from build123d import *

# Parameters (mm, degrees)
SKETCH1_R             = 22.5
BOSS_EXTRUDE1_DEPTH   = 75
BOSS_EXTRUDE1_2_DEPTH = 75
SKETCH1_W             = 45
SKETCH1_H             = 45
BOSS_EXTRUDE1_3_DEPTH = 75
SKETCH2_W             = 218.297343906
SKETCH2_H             = 67.055865706
BOSS_EXTRUDE2_DEPTH   = 3


with BuildPart() as part:
    # Sketch1 → Boss-Extrude1 (new body)
    with BuildSketch(Plane.XY):
        with Locations((72.5, 0)):
            Circle(SKETCH1_R)
    extrude(amount=BOSS_EXTRUDE1_DEPTH)



with BuildPart() as body_2:
    # Sketch1 → Boss-Extrude1 2 (new body)
    with BuildSketch(Plane.XY):
        Polygon((-22.5, -12.990381057), (0, 25.980762114), (22.5, -12.990381057), align=None)
    extrude(amount=BOSS_EXTRUDE1_2_DEPTH)


with BuildPart() as body_3:
    # Sketch1 → Boss-Extrude1 3 (new body)
    with BuildSketch(Plane.XY):
        with Locations((-70, 0)):
            Rectangle(SKETCH1_W, SKETCH1_H)
    extrude(amount=BOSS_EXTRUDE1_3_DEPTH)


with BuildPart() as part_1:
    add(part.part)

    add(body_2.part)  # Boss-Extrude2 merges body 2

    add(body_3.part)  # Boss-Extrude2 merges body 3
    # Sketch2 → Boss-Extrude2 (add)
    with BuildSketch(Plane.XY.offset(75)):
        Rectangle(SKETCH2_W, SKETCH2_H)
    extrude(amount=BOSS_EXTRUDE2_DEPTH)


solid = part_1.part
Can you work these out from the model? Positions are in its coordinate system, mm. A direction names the side the tool comes from. Coordinates: 2 decimals unless noted, no trailing zeros. Loops run counter-clockwise (first coordinate to the right, second up) from the corner with the lowest first, then second, coordinate; pieces in that order, holes last. Notation, with made-up numbers: M 30.5,-36 L 78.5,-36 A28 ccw 78.5,0 Z; hole C 84,-3.75 d1. An arc over 180 degrees is marked long. Return JSON: item names as keys, results as strings. Group by question number.
Item 1: Imagine slicing it at D-D (x = 10.5). Please give me the cut outline in (y, z), and give its area (3 significant figures).
Item 2: If I drill on L1, parallel to X at y = 5.5, z = 35; L2, parallel to X at y = -9.5, z = 47; L3, parallel to Z at x = -31.5, y = -6, over which ranges is the centre line in solid material (lowest first)? Write a range as from..to.
Item 3: I'm going to push flat-ended pins straight in: pin 1 Ø10 at (y, z) = (12.5, 49) entering from -X; pin 2 Ø12 at (x, z) = (47, 62) entering from -Y (3 decimals); pin 3 Ø3 at (y, z) = (22, 36) entering from +X; pin 4 Ø10 at (x, z) = (42.5, 37.5) entering from +Y. Where does each tip first touch, or does it pass through?
Item 4: On a 3-axis mill with a long thin cutter (end or side, diameter ignored), from which of +Z, -Z, +X, -X, +Y, -Y can I reach the whole of each face in a straight line? I mean faces 4 (the flat face through (-70, 22.5, 37)), 5 (the flat face through (-47.5, 0, 37)), 6 (the cylindrical face through (50.02, 0.99, 36.98)), 7 (the flat face through (11.09, 6.77, 36.98)), 8 (the flat face through (-70, -22.5, 37)). Say none if no direction works.
Item 5: Imagine slicing it at A-A (z = 30.5). Please give me the cut outline in (x, y), and give its area (3 significant figures).
Item 6: Imagine slicing it at C-C (x = 72.5). Please give me the cut outline in (y, z), and give its area (3 significant figures).
Item 7: Imagine slicing it at B-B (y = 0). Please give me the cut outline in (x, z).
Item 8: Thinking about a two-plate mould opening in X: for faces 1 (the flat face through (72, 0, 0)), 2 (the flat face through (-92.5, 0, 37)), 3 (the flat face through (-11.41, 6.22, 36.98)), which applies, released by +X, released by -X, zero draft, split by the parting line, or undercut?
Verdict:
{
 "1": {"outline": "M -33.53,75 L -12.99,75 L -12.99,0 L 7.79,0 L 7.79,75 L 33.53,75 L 33.53,78 L -33.53,78 Z", "area": "1,760 mm^2"},
 "2": {"L1": "x = -92.5..-47.5, -11.82..11.82, 50.68..94.32", "L2": "x = -92.5..-47.5, -20.48..20.48, 52.1..92.9", "L3": "z = 75..78"},
 "3": {"pin 1": "stops at x = -92.5", "pin 2": "stops at y = -11.225", "pin 3": "stops at x = 81.77", "pin 4": "passes through"},
 "4": {"face 4": "-Z, -X, +Y", "face 5": "-Z, +Y, -Y", "face 6": "-Z", "face 7": "-Z, +Y", "face 8": "-Z, +X, -X, -Y"},
 "5": {"outline": "M -92.5,-22.5 L -47.5,-22.5 L -47.5,22.5 L -92.5,22.5 Z; M -22.5,-12.99 L 22.5,-12.99 L 0,25.98 Z; C 72.5,0 d45", "area": "4,490 mm^2"},
 "6": {"outline": "M -33.53,75 L -22.5,75 L -22.5,0 L 22.5,0 L 22.5,75 L 33.53,75 L 33.53,78 L -33.53,78 Z", "area": "3,580 mm^2"},
 "7": {"outline": "M -109.15,75 L -92.5,75 L -92.5,0 L -47.5,0 L -47.5,75 L -15,75 L -15,0 L 15,0 L 15,75 L 50,75 L 50,0 L 95,0 L 95,75 L 109.15,75 L 109.15,78 L -109.15,78 Z"},
 "8": {"face 1": "zero draft", "face 2": "released by -X", "face 3": "undercut"}
}
